from build123d import *

# Parameters (mm, degrees)
SKETCH2_R           = 125
BOSS_EXTRUDE1_DEPTH = 1.5
SKETCH3_W           = 3
SKETCH3_H           = 19
CUT_EXTRUDE1_DEPTH  = 177.783059143
SKETCH4_R           = 1.8
CUT_EXTRUDE2_DEPTH  = 177.783059143
CUT_EXTRUDE5_DEPTH  = 177.783059143
CIRPATTERN2_COUNT   = 3


with BuildPart() as part:
    # Sketch2 → Boss-Extrude1 (new body)
    with BuildSketch(Plane(origin=(0, 0, 0), x_dir=(1, 0, 0), z_dir=(0, 1, 0))):
        with Locations(Location((0, 0, 0), (0, 0, 270))):
            Circle(SKETCH2_R)
    extrude(amount=BOSS_EXTRUDE1_DEPTH)

    # Sketch3 → Cut-Extrude1 (cut, through all)
    with BuildSketch(Plane(origin=(0, 1.5, 0), x_dir=(1, 0, 0), z_dir=(0, 1, 0))):
        with Locations((-268.691654721, -368.173324402)):
            Rectangle(SKETCH3_W, SKETCH3_H)
        Polygon((31.312, -98.125219266), (35.122688127, -96.909219266), (40.898688127, -115.009987868), (37.088, -116.225987868), align=None)
        Polygon((-37.088, -116.225987868), (-31.312, -98.125219266), (-35.122688127, -96.909219266), (-40.898688127, -115.009987868), align=None)
        Polygon((-82.110658074, 90.23214411), (-69.322932636, 76.179597076), (-66.364501682, 78.8717498), (-79.15222712, 92.924296834), align=None)
        Polygon((-100.634932636, 21.94562219), (-101.487189809, 18.037469466), (-120.050915246, 22.085691035), (-119.198658074, 25.993843759), align=None)
        Polygon((119.198658074, 25.993843759), (100.634932636, 21.94562219), (101.487189809, 18.037469466), (120.050915246, 22.085691035), align=None)
        Polygon((69.322932636, 76.179597076), (66.364501682, 78.8717498), (79.15222712, 92.924296834), (82.110658074, 90.23214411), align=None)
    extrude(amount=-CUT_EXTRUDE1_DEPTH, mode=Mode.SUBTRACT)

    # Sketch4 → Cut-Extrude2 (cut, through all)
    with BuildSketch(Plane(origin=(0, 1.5, 0), x_dir=(1, 0, 0), z_dir=(0, 1, 0))):
        with Locations(Location((0, 85, 0), (0, 0, 270))):
            Circle(SKETCH4_R)
        with Locations(Location((73.612159322, -42.5, 0), (0, 0, 270))):
            Circle(SKETCH4_R)
        with Locations(Location((-73.612159322, -42.5, 0), (0, 0, 270))):
            Circle(SKETCH4_R)
    extrude(amount=-CUT_EXTRUDE2_DEPTH, mode=Mode.SUBTRACT)

    # Sketch6 → Cut-Extrude5 (cut, through all)
    with BuildSketch(Plane(origin=(0, 1.5, 0), x_dir=(1, 0, 0), z_dir=(0, 1, 0))):
        Polygon((-55.992533724, -149.153029157), (-67.424598105, -145.505029157), (-48.541440634, -86.329187076), (-37.109376254, -89.977187076), align=None)
        Polygon((67.424598105, -145.505029157), (48.541440634, -86.329187076), (37.109376254, -89.977187076), (55.992533724, -149.153029157), align=None)
    cut_extrude5 = extrude(amount=-CUT_EXTRUDE5_DEPTH, mode=Mode.SUBTRACT)

    # CirPattern2: Cut-Extrude5 ×3 about axis
    cirpattern2_axis = Axis((0, 0, 0), (0, 1, 0))
    for i in range(1, CIRPATTERN2_COUNT):
        add(cut_extrude5.rotate(cirpattern2_axis, i * 360 / CIRPATTERN2_COUNT), mode=Mode.SUBTRACT)


solid = part.part
For this review, take the finished solid that the model builds, in its own axes (mm). A direction names the side the tool comes from. Round coordinates to 2 decimals unless told otherwise and drop trailing zeros. Write each loop counter-clockwise with the first axis right and the second up, starting at its lowest first coordinate (ties: lowest second). Pieces come first, ordered by that corner, then holes. Notation, with made-up numbers: M 26.25,25.5 L 46.25,25.5 A20 cw 46.25,53.5 Z; hole C 64,-34.75 d11. An arc over 180 degrees is marked long. Write item = value, one per line. Start each with the question number.
(1) We need section A-A (z = 107.5). Give the boundary of the cut face in (x, y).
(2) We need section B-B (y = 0.4). Give the number of separate pieces and of enclosed holes in the cut face, then the cut area to 3 significant figures.
(3) For line 1 along X through (y, z) = (0.9, 42.5); line 2 along X through (y, z) = (0.2, -90.5) (3 decimals); line 3 along Z through (x, y) = (66, 0.1), list the stretches that pass through material, from the lowest coordinate up.
(4) Clearance check with a flat-ended pin moving along its axis: pin 1 Ø3 at (x, z) = (0, -85) entering from +Y. State where the tip first meets the part, or that it passes through.
(5) We need section C-C (z = 56.5). Give the boundary of the cut face in (x, y), then the cut area to 3 significant figures.
(6) For faces 1 (the face through (-68.57, 0.76, -87.24)), 2 (the face through (-107.93, 0.74, -63.06)), 3 (the face through (-52.61, 0.76, 99.08)), 4 (the face through (109.841, 0.76, -15.765)), 5 (the face through (-109.841, 0.76, -15.765)), list the 3-axis set-ups (+Z, -Z, +X, -X, +Y, -Y) from which the entire face can be reached by the end or side of a thin tool; tool diameter is ignored.
(7) The part is to be moulded in two halves that separate along Z. For faces 6 (the face through (2, 0, -2)), 7 (the face through (108.58, 0.74, -61.93)), 8 (the face through (68.57, 0.76, -87.24)), say which applies: +Z half, -Z half, draft (parallel to the pull), parting line (faces both ways), or undercut.
Results found:
q1.outline = M -63.79,0 L -55.3,0 L -55.3,1.5 L -63.79,1.5 Z; M -42.7,0 L -38.5,0 L -38.5,1.5 L -42.7,1.5 Z; M -34.3,0 L 34.3,0 L 34.3,1.5 L -34.3,1.5 Z; M 38.5,0 L 42.7,0 L 42.7,1.5 L 38.5,1.5 Z; M 55.3,0 L 63.79,0 L 63.79,1.5 L 55.3,1.5 Z
q2.separate_pieces = 1
q2.enclosed_holes = 9
q2.area = 46,600 mm²
q3.line_1 = -117.55 to -75.41, -71.81 to 71.81, 75.41 to 117.55
q3.line_2 = -86.225 to -81.816, -76.946 to -71.538, -55.313 to 55.313, 71.538 to 76.946, 81.816 to 86.225
q3.line_3 = -106.16 to -102.24, -84.41 to 106.16
q4.pin_1 = through
q5.outline = M -111.5,0 L 111.5,0 L 111.5,1.5 L -111.5,1.5 Z
q5.area = 335 mm²
q6.face_1 = +Y, -Y
q6.face_2 = -Z, -X, +Y, -Y
q6.face_3 = +Z, +Y, -Y
q6.face_4 = +X, +Y, -Y
q6.face_5 = -X, +Y, -Y
q7.face_6 = draft
q7.face_7 = -Z half
q7.face_8 = undercut
